from build123d import *

# Parameters (mm, degrees)
SKETCH001_W  = 68
SKETCH001_H  = 72.5
PAD001_DEPTH = 18
SKETCH002_W  = 71.665652
SKETCH002_H  = 18.549143
PAD002_DEPTH = 10
SKETCH_W     = 80.745956
SKETCH_H     = 20.815728
SKETCH_R     = 1.75
PAD_DEPTH    = 3


with BuildPart() as pad001:
    # Sketch001 → Pad001 (new body)
    with BuildSketch(Plane.XY):
        with Locations((0, 1.520855)):
            Rectangle(SKETCH001_W, SKETCH001_H)
    extrude(amount=PAD001_DEPTH)


with BuildPart() as pad002:
    # Sketch002 → Pad002 (new body)
    with BuildSketch(Plane.XZ.offset(-15)):
        with Locations((0, 10.925129)):
            Rectangle(SKETCH002_W, SKETCH002_H)
    extrude(amount=PAD002_DEPTH)


with BuildPart() as cut:
    # Sketch → Pad (new body)
    with BuildSketch(Plane.XY):
        with Locations((0, 4.542604)):
            Rectangle(SKETCH_W, SKETCH_H)
        with Locations((-37, 0)):
            Circle(SKETCH_R, mode=Mode.SUBTRACT)
        with Locations((37, 0)):
            Circle(SKETCH_R, mode=Mode.SUBTRACT)
    extrude(amount=PAD_DEPTH)

    # Fusion: union Pad002
    add(pad002.part)

    # Cut: cut Pad001
    add(pad001.part, mode=Mode.SUBTRACT)


solid = cut.part
Input: part model. Units: mm. Frame: model coordinates. A direction names the side the tool comes from. Coordinates: 2 decimals unless noted, no trailing zeros. Loops run counter-clockwise (first coordinate to the right, second up) from the corner with the lowest first, then second, coordinate; pieces in that order, holes last.
Q1. Cut plane B-B (y = 3). Output: boundary loops of the cut face in (x, z).
Q2. Material intervals for line 1 (Y direction, x = 37, z = 0.6); line 2 (X direction, y = 13.75, z = 13.75); line 3 (Z direction, x = -10, y = 6), sorted ascending.
Q3. Cut plane C-C (y = 10). Output: boundary loops of the cut face in (x, z).
Q4. Cut plane A-A (x = -37). Output: boundary loops of the cut face in (y, z).
Q5. Set-up query: faces 4 (the face through (0, 10, 18)), 5 (the face through (0, 5, 19)), 6 (the face through (37, -5.865, 1)). Return all of +Z, -Z, +X, -X, +Y, -Y with unobstructed straight access to the full face (end or side cutting, diameter ignored); none if empty.
Q6. Draft query along X for faces 1 (the face through (34, 9, 7)), 2 (the face through (40.373, 4, 1)), 3 (the face through (-38, 5, 3)). Return one class per face: +X half, -X half, draft (parallel to the pull), parting line (faces both ways), or undercut.
Q7. Contact query for flat-ended pins moving along their axis: pin 1 (8 mm diameter, centred on y = 10.5, z = 12.5, fed in from +X); pin 2 (3.5 mm diameter, centred on x = 38.5, z = 2, fed in from +Y); pin 3 (6 mm diameter, centred on x = 2, y = 7, fed in from -Z). Output: stop coordinate, or through.
Working result:
1. outline: (-40.37, 0) - (-34, 0) - (-34, 3) - (-40.37, 3) - close; (34, 0) - (40.37, 0) - (40.37, 3) - (34, 3) - close
2. line 1: y = -5.87 to -1.75, 1.75 to 14.95
2. line 2: x = -35.83 to -34, 34 to 35.83
2. line 3: z = 18 to 20.2
3. outline: (-40.37, 0) - (-34, 0) - (-34, 18) - (34, 18) - (34, 0) - (40.37, 0) - (40.37, 3) - (35.83, 3) - (35.83, 20.2) - (-35.83, 20.2) - (-35.83, 3) - (-40.37, 3) - close
4. outline: (-5.87, 0) - (-1.75, 0) - (-1.75, 3) - (-5.87, 3) - close; (1.75, 0) - (14.95, 0) - (14.95, 3) - (1.75, 3) - close
5. face 4: -Z, +Y, -Y
5. face 5: +Z, +X, -X, -Y
5. face 6: +Z, -Z, +X, -X, -Y
6. face 1: undercut
6. face 2: +X half
6. face 3: draft
7. pin 1: stops at x = 35.83
7. pin 2: stops at y = 14.95
7. pin 3: stops at z = 18
